Could you check a few things on this model? Use its own coordinates, in mm. A direction names the side the tool comes from. Round coordinates to 2 decimals unless told otherwise and drop trailing zeros. Write each loop counter-clockwise with the first axis right and the second up, starting at its lowest first coordinate (ties: lowest second). Pieces come first, ordered by that corner, then holes. Notation, with made-up numbers: (29.5, 51) -> (61.5, 51) arc R35 cw to (61.5, 84) -> close; hole circle Ø10 at (77.5, 15). An arc over 180 degrees is marked (long way). Answer as CSV lines item,"result". Start each with the question number.
Q1. Imagine slicing it at C-C on z = -8. Please give me the cut outline in (x, y), and give its area (3 significant figures).
Q2. If I drill on line 1 (X direction, y = 2.45, z = -8); line 2 (X direction, y = 1.9, z = -30); line 3 (Z direction, x = 9, y = 0.7), over which ranges is the centre line in solid material (lowest first)? Write a range as [from, to].
Q3. Imagine slicing it at D-D on z = 43.5. Please give me the cut outline in (x, y), and give its area (3 significant figures).
Q4. Will these pins go through, and if not, where does the flat tip stop? pin 1 Ø2.5 at (x, z) = (0, 72.2) entering from +Y; pin 2 Ø1.5 at (y, z) = (1, 55.5) entering from -X; pin 3 Ø0.9 at (y, z) = (1, 0.5) entering from -X; pin 4 Ø1.5 at (y, z) = (1.5, 2.5) entering from +X.
Q5. Imagine slicing it at B-B on x = 0. Please give me the cut outline in (y, z), and give its area (3 significant figures).
Q6. If we mould it in two halves opening along Z, with no side actions, what happens to faces 1 (the flat face through (-15, 1, -36.273)), 2 (the cylindrical face through (15.655, 1.479, -7.079)), 3 (the flat face through (14.5, 1, 71))? For each: pulls with the +Z half, pulls with the -Z half, needs draft (parallel to the pull), parting line crosses it, or undercut.
Q7. Imagine slicing it at A-A on z = 27. Please give me the cut outline in (x, y), and give its area (3 significant figures).
Q8. For faces 4 (the flat face through (-20.778, 1.479, 22.662)), 5 (the flat face through (0, 1, -35)), 6 (the flat face through (-21.885, 1, 29)), 7 (the cylindrical face through (-10.196, 1.521, 33.289)), which set-ups out of +Z, -Z, +X, -X, +Y, -Y let a thin tool reach every point of the face, with its end or its side?
from build123d import *

# Parameters (mm, degrees)
SKETCH_1_R          = 1.5
SKETCH_1_R_2        = 1.25
SKETCH_1_W          = 24
SKETCH_1_H          = 66.5
EXTRUDE_1_DEPTH     = 3
FILLET_1_R          = 1.5
CUT_EXTRUDE_1_DEPTH = 3
FILLET_2_R          = 1
FILLET_3_R          = 1.5
FILLET_4_R          = 2
FILLET_5_R          = 2
FILLET_6_R          = 6


with BuildPart() as part:
    # 草图1 → 凸台-拉伸1 (new body)
    with BuildSketch(Plane(origin=(0, 0, 0), x_dir=(1, 0, 0), z_dir=(0, 1, 0))):
        Polygon((10.04233564, 35), (-10.04233564, 35), (-12.523742682, 36.273217412), (-19.001684764, 36.273217412), (-23.015493308, 30.5), (-19.695655938, 22.877483708), (-19.695655938, -20.552984489), (-21.884751354, -24.819370363), (-21.884751354, -32.255531362), (-14.5, -68.123136609), (-14.5, -75.2), (14.5, -75.2), (14.5, -68.123136609), (21.884751354, -32.255531362), (21.884751354, -24.819370363), (19.695655938, -20.552984489), (19.695655938, 22.877483708), (23.015493308, 30.5), (19.001684764, 36.273217412), (12.523742682, 36.273217412), align=None)
        with Locations(Location((-18, 30, 0), (0, 0, 270))):
            Circle(SKETCH_1_R, mode=Mode.SUBTRACT)
        with Locations(Location((18, 30, 0), (0, 0, 270))):
            Circle(SKETCH_1_R, mode=Mode.SUBTRACT)
        with Locations(Location((18, -30, 0), (0, 0, 270))):
            Circle(SKETCH_1_R, mode=Mode.SUBTRACT)
        with Locations(Location((-18, -30, 0), (0, 0, 270))):
            Circle(SKETCH_1_R, mode=Mode.SUBTRACT)
        with Locations(Location((0, -72.2, 0), (0, 0, 270))):
            Circle(SKETCH_1_R, mode=Mode.SUBTRACT)
        with Locations(Location((-10, -43.5, 0), (0, 0, 270))):
            Circle(SKETCH_1_R, mode=Mode.SUBTRACT)
        with Locations(Location((10, -43.5, 0), (0, 0, 90))):
            Circle(SKETCH_1_R, mode=Mode.SUBTRACT)
        with Locations(Location((-16.5, 8, 0), (0, 0, 270))):
            Circle(SKETCH_1_R_2, mode=Mode.SUBTRACT)
        with Locations(Location((16.5, 8, 0), (0, 0, 90))):
            Circle(SKETCH_1_R_2, mode=Mode.SUBTRACT)
        with Locations((0, -1.75)):
            Rectangle(SKETCH_1_W, SKETCH_1_H, mode=Mode.SUBTRACT)
    extrude(amount=EXTRUDE_1_DEPTH)

    # 圆角1
    fillet_1_edges = [part.edges().sort_by_distance(p)[0] for p in [
        (12, 1.5, -31.5),
        (-12, 1.5, -31.5),
    ]]
    fillet(fillet_1_edges, radius=FILLET_1_R)

    # 草图2 → 切除-拉伸1 (cut)
    with BuildSketch(Plane(origin=(0, 3, 0), x_dir=(1, 0, 0), z_dir=(0, 1, 0))):
        with BuildLine():
            ThreePointArc((-16.09935509, -33.519594994), (-17.804419777, -33.995215686), (-19.547787148, -33.688408186))
            Line((-19.547787148, -33.688408186), (-11.5, -72.77636643))
            Line((-11.5, -72.77636643), (-11.5, -46.098076211))
            ThreePointArc((-11.5, -46.098076211), (-12.930484116, -44.14207698), (-12.448919233, -41.767142652))
            Line((-12.448919233, -41.767142652), (-16.09935509, -33.519594994))
        make_face()
        with BuildLine():
            ThreePointArc((-7.401923789, -45), (-7.878679656, -45.621320344), (-8.5, -46.098076211))
            Line((-8.5, -46.098076211), (-8.5, -72.142731986))
            Line((-8.5, -72.142731986), (-2.999453346, -72.142731986))
            ThreePointArc((-2.999453346, -72.142731986), (-2.43284555, -70.444647463), (-1, -69.371572875))
            Line((-1, -69.371572875), (-1, -45))
            Line((-1, -45), (-7.401923789, -45))
        make_face()
        with BuildLine():
            Line((7.401923789, -45), (1, -45))
            Line((1, -45), (1, -69.371572875))
            ThreePointArc((1, -69.371572875), (2.43284555, -70.444647463), (2.999453346, -72.142731986))
            Line((2.999453346, -72.142731986), (8.5, -72.142731986))
            Line((8.5, -72.142731986), (8.5, -46.098076211))
            ThreePointArc((8.5, -46.098076211), (7.878679656, -45.621320344), (7.401923789, -45))
        make_face()
        with BuildLine():
            ThreePointArc((12.448919233, -41.767142652), (12.930484116, -44.14207698), (11.5, -46.098076211))
            Line((11.5, -46.098076211), (11.5, -72.77636643))
            Line((11.5, -72.77636643), (19.547787148, -33.688408186))
            ThreePointArc((19.547787148, -33.688408186), (17.804419777, -33.995215686), (16.09935509, -33.519594994))
            Line((16.09935509, -33.519594994), (12.448919233, -41.767142652))
        make_face()
    extrude(amount=-CUT_EXTRUDE_1_DEPTH, mode=Mode.SUBTRACT)

    # 圆角2
    fillet_2_edges = [part.edges().sort_by_distance(p)[0] for p in [
        (-11.5, 1.5, 72.77636643),
        (-19.547787148, 1.5, 33.688408186),
        (-16.09935509, 1.5, 33.519594994),
        (19.547787148, 1.5, 33.688408186),
        (11.5, 1.5, 72.77636643),
        (16.09935509, 1.5, 33.519594994),
    ]]
    fillet(fillet_2_edges, radius=FILLET_2_R)

    # 圆角3
    fillet_3_edges = [part.edges().sort_by_distance(p)[0] for p in [
        (8.5, 1.5, 46.098076211),
        (8.5, 1.5, 72.142731986),
        (2.999453346, 1.5, 72.142731986),
        (1, 1.5, 69.371572875),
        (1, 1.5, 45),
        (7.401923789, 1.5, 45),
        (-1, 1.5, 69.371572875),
        (-2.999453346, 1.5, 72.142731986),
        (-8.5, 1.5, 72.142731986),
        (-8.5, 1.5, 46.098076211),
        (-7.401923789, 1.5, 45),
        (-1, 1.5, 45),
    ]]
    fillet(fillet_3_edges, radius=FILLET_3_R)

    # 圆角4
    fillet_4_edges = [part.edges().sort_by_distance(p)[0] for p in [
        (-12.448919233, 1.5, 41.767142652),
        (-11.5, 1.5, 46.098076211),
        (11.5, 1.5, 46.098076211),
        (12.448919233, 1.5, 41.767142652),
    ]]
    fillet(fillet_4_edges, radius=FILLET_4_R)

    # 圆角5
    fillet_5_edges = [part.edges().sort_by_distance(p)[0] for p in [
        (-12.523742682, 1.5, -36.273217412),
        (-10.04233564, 1.5, -35),
        (10.04233564, 1.5, -35),
        (12.523742682, 1.5, -36.273217412),
        (19.001684764, 1.5, -36.273217412),
        (23.015493308, 1.5, -30.5),
        (19.695655938, 1.5, -22.877483708),
        (19.695655938, 1.5, 20.552984489),
        (21.884751354, 1.5, 24.819370363),
        (21.884751354, 1.5, 32.255531362),
        (14.5, 1.5, 68.123136609),
        (14.5, 1.5, 75.2),
        (-14.5, 1.5, 75.2),
        (-14.5, 1.5, 68.123136609),
        (-21.884751354, 1.5, 32.255531362),
        (-21.884751354, 1.5, 24.819370363),
        (-19.695655938, 1.5, 20.552984489),
        (-19.695655938, 1.5, -22.877483708),
        (-23.015493308, 1.5, -30.5),
        (-19.001684764, 1.5, -36.273217412),
    ]]
    fillet(fillet_5_edges, radius=FILLET_5_R)

    # 圆角6
    fillet_6_edges = [part.edges().sort_by_distance(p)[0] for p in [
        (12, 1.5, 35),
        (-12, 1.5, 35),
    ]]
    fillet(fillet_6_edges, radius=FILLET_6_R)


solid = part.part
Checks:
1,outline,"(-19.7, 0) -> (-17.75, 0) -> (-17.75, 3) -> (-19.7, 3) -> close; (-15.25, 0) -> (-12, 0) -> (-12, 3) -> (-15.25, 3) -> close; (12, 0) -> (15.25, 0) -> (15.25, 3) -> (12, 3) -> close; (17.75, 0) -> (19.7, 0) -> (19.7, 3) -> (17.75, 3) -> close"
1,area,"31.2 mm^2"
2,line 1,"[-19.7, -17.75], [-15.25, -12], [12, 15.25], [17.75, 19.7]"
2,line 2,"[-22.72, -19.5], [-16.5, -12], [12, 16.5], [19.5, 22.72]"
2,line 3,"[-35, -31.5], [34.2, 42.38], [44.62, 75.2]"
3,outline,"(-19.57, 0) -> (-17.53, 0) -> (-17.53, 3) -> (-19.57, 3) -> close; (-13, 0) -> (-11.5, 0) -> (-11.5, 3) -> (-13, 3) -> close; (-8.5, 0) -> (8.5, 0) -> (8.5, 3) -> (-8.5, 3) -> close; (11.5, 0) -> (13, 0) -> (13, 3) -> (11.5, 3) -> close; (17.53, 0) -> (19.57, 0) -> (19.57, 3) -> (17.53, 3) -> close"
3,area,"72.3 mm^2"
4,pin 1,"through"
4,pin 2,"x = -17.25"
4,pin 3,"x = -19.7"
4,pin 4,"x = 19.7"
5,outline,"(0, -35) -> (3, -35) -> (3, -31.5) -> (0, -31.5) -> close; (0, 35) -> (3, 35) -> (3, 70.7) -> (0, 70.7) -> close; (0, 73.7) -> (3, 73.7) -> (3, 75.2) -> (0, 75.2) -> close"
5,area,"122 mm^2"
6,face 1,"pulls with the -Z half"
6,face 2,"undercut"
6,face 3,"needs draft"
7,outline,"(-21.88, 0) -> (-12, 0) -> (-12, 3) -> (-21.88, 3) -> close; (12, 0) -> (21.88, 0) -> (21.88, 3) -> (12, 3) -> close"
7,area,"59.3 mm^2"
8,face 4,"-X, +Y, -Y"
8,face 5,"-Z, +Y, -Y"
8,face 6,"+Z, -X, +Y, -Y"
8,face 7,"+Y, -Y"
